CAD build for the part. Positions are in the model's coordinates, mm. A direction names the side the tool comes from. Give positions to 0.01 mm unless a question says otherwise; leave off trailing zeros. Write each loop counter-clockwise with the first axis right and the second up, starting at its lowest first coordinate (ties: lowest second). Pieces come first, ordered by that corner, then holes. Notation, with made-up numbers: (27.25, -2.5) -> (67.25, -2.5) arc R29 cw to (67.25, 20.5) -> close; hole circle Ø9 at (56, 51). An arc over 180 degrees is marked (long way). Use one line per item in the form item = value. Start each with the question number.
from build123d import *

# Parameters (mm, degrees)
BOSS_EXTRUDE1_DEPTH = 20
SKETCH2_R           = 3.25
CUT_EXTRUDE1_DEPTH  = 55.919366752
SKETCH3_R           = 9.1
CUT_EXTRUDE2_DEPTH  = 2
SKETCH4_R           = 1.7
CUT_EXTRUDE3_DEPTH  = 55.919366752
SKETCH5_R           = 1.7
CUT_EXTRUDE4_DEPTH  = 53.677895109
RIB26_REACH         = 46.958
SKETCH15_WALL_W     = 134.175527088
SKETCH15_WALL_H     = 10


with BuildPart() as part:
    # Sketch1 → Boss-Extrude1 (new, symmetric)
    with BuildSketch(Plane(origin=(0, 0, 0), x_dir=(0, 0, -1), z_dir=(1, 0, 0))):
        Polygon((24.929590164, 27.161885246), (24.929590164, -27.838114754), (-29.090409836, -27.838114754), (-29.090409836, -14.908114754), (10.909590164, -14.908114754), (10.909590164, 27.161885246), align=None)
    extrude(amount=BOSS_EXTRUDE1_DEPTH, both=True)

    # Sketch2 → Cut-Extrude1 (cut, through all)
    with BuildSketch(Plane(origin=(0, -14.908114754, 0), x_dir=(1, 0, 0), z_dir=(0, 1, 0))):
        with Locations(Location((0, -9.090409836, 0), (0, 0, 270))):
            Circle(SKETCH2_R)
    extrude(amount=-CUT_EXTRUDE1_DEPTH, mode=Mode.SUBTRACT)

    # Sketch3 → Cut-Extrude2 (cut)
    with BuildSketch(Plane(origin=(0, -14.908114754, 0), x_dir=(1, 0, 0), z_dir=(0, 1, 0))):
        with Locations(Location((0, -9.090409836, 0), (0, 0, 270))):
            Circle(SKETCH3_R)
    extrude(amount=-CUT_EXTRUDE2_DEPTH, mode=Mode.SUBTRACT)

    # Sketch4 → Cut-Extrude3 (cut, through all)
    with BuildSketch(Plane(origin=(0, -14.908114754, 0), x_dir=(1, 0, 0), z_dir=(0, 1, 0))):
        with Locations(Location((0, 1.909590164, 0), (0, 0, 270))):
            Circle(SKETCH4_R)
        with Locations(Location((11, -9.090409836, 0), (0, 0, 270))):
            Circle(SKETCH4_R)
        with Locations(Location((0, -20.090409836, 0), (0, 0, 270))):
            Circle(SKETCH4_R)
        with Locations(Location((-11, -9.090409836, 0), (0, 0, 270))):
            Circle(SKETCH4_R)
    extrude(amount=-CUT_EXTRUDE3_DEPTH, mode=Mode.SUBTRACT)

    # Sketch5 → Cut-Extrude4 (cut, through all)
    with BuildSketch(Plane.XY.offset(-10.909590164)):
        with Locations((-10, 16.126885246)):
            Circle(SKETCH5_R)
        with Locations((10, 16.126885246)):
            Circle(SKETCH5_R)
        with Locations((10, -3.873114754)):
            Circle(SKETCH5_R)
        with Locations((-10, -3.873114754)):
            Circle(SKETCH5_R)
    extrude(amount=-CUT_EXTRUDE4_DEPTH, mode=Mode.SUBTRACT)

    # Sketch15 wall → Rib26 (add, up to next)
    with BuildSketch(Plane(origin=(0, 6.126885246, -8.909590164), x_dir=(0, -0.995510349515, 0.094652754886), z_dir=(0, 0.094652754886, 0.995510349515)), mode=Mode.PRIVATE) as rib26_sk1:
        Rectangle(SKETCH15_WALL_W, SKETCH15_WALL_H)
    rib26_tool1 = extrude(rib26_sk1.sketch, amount=-RIB26_REACH, mode=Mode.PRIVATE) - part.part
    add(rib26_tool1.solids().sort_by_distance((0, 6.126885246, -8.909590164))[0])


solid = part.part
1) 3-axis set-ups, long thin cutter, end or side, ignore diameter. For faces 4 (the face through (-12.03, -21.28, 7.74)), 5 (the face through (13, 6, -10.91)), 6 (the face through (-12, 6, -10.91)), 7 (the face through (-4, -16.908, 9)), 8 (the face through (0, -27.838, 2)): which of +Z, -Z, +X, -X, +Y, -Y reach the whole face in a straight line?
2) Cut at B-B (z = 21). Give the cut face in (x, y).
3) Cut at C-C (y = -21.5). Give the cut face in (x, z), and give its area (3 significant figures).
4) Two-plate mould, pull along X, no slides. Class faces 1 (the face through (0, 0, -24.93)), 2 (the face through (9.779, 17.812, -17.821)), 3 (the face through (-5, 2, -10)): released by +X, released by -X, zero draft, split by the parting line, or undercut.
5) Cut at D-D (z = -16). Give the cut face in (x, y).
6) Wall check: line 1 along Y through (x, z) = (10.5, 16); line 2 along Y through (x, z) = (8, 12); line 3 along Z through (x, y) = (-3, -24.5). Give the ranges that are in metal, low to high. Write a range as from..to.
7) Cut at A-A (x = 0). Give the cut face in (y, z), and give its area (3 significant figures).
8) Pin check, flat tips, straight feed: pin 1 (3 mm diameter, centred on y = 10, z = -9, fed in from -X); pin 2 (4.5 mm diameter, centred on x = 10, y = 16.13, fed in from +Z); pin 3 (14.5 mm diameter, centred on x = 4, z = 7, fed in from +Y). Stop position of each tip, or through.
Final values:
q1.face_4 = +Y, -Y
q1.face_5 = +Z, +X, +Y
q1.face_6 = +Z, -X, +Y
q1.face_7 = +Y
q1.face_8 = +Z, -Z, +X, -X, -Y
q2.outline = (-20, -27.84) -> (-1.44, -27.84) -> (-1.44, -14.91) -> (-20, -14.91) -> close; (1.44, -27.84) -> (20, -27.84) -> (20, -14.91) -> (1.44, -14.91) -> close
q3.outline = (-20, -24.93) -> (20, -24.93) -> (20, 29.09) -> (-20, 29.09) -> close; hole circle Ø3.4 at (-11, 9.09); hole circle Ø6.5 at (0, 9.09); hole circle Ø3.4 at (0, -1.91); hole circle Ø3.4 at (0, 20.09); hole circle Ø3.4 at (11, 9.09)
q3.area = 2,090 mm^2
q4.face_1 = zero draft
q4.face_2 = undercut
q4.face_3 = released by -X
q5.outline = (-20, -27.84) -> (20, -27.84) -> (20, 27.16) -> (-20, 27.16) -> close; hole circle Ø3.4 at (-10, -3.87); hole circle Ø3.4 at (-10, 16.13); hole circle Ø3.4 at (10, -3.87); hole circle Ø3.4 at (10, 16.13)
q6.line_1 = -27.84..-14.91
q6.line_2 = -27.84..-16.91
q6.line_3 = -24.93..7.84, 10.34..29.09
q7.outline = (-27.84, -24.93) -> (27.16, -24.93) -> (27.16, -10.91) -> (-14.91, -6.91) -> (-14.91, -3.61) -> (-27.84, -3.61) -> close; (-27.84, -0.21) -> (-14.91, -0.21) -> (-14.91, -0.01) -> (-16.91, -0.01) -> (-16.91, 5.84) -> (-27.84, 5.84) -> close; (-27.84, 12.34) -> (-16.91, 12.34) -> (-16.91, 18.19) -> (-14.91, 18.19) -> (-14.91, 18.39) -> (-27.84, 18.39) -> close; (-27.84, 21.79) -> (-14.91, 21.79) -> (-14.91, 29.09) -> (-27.84, 29.09) -> close
q7.area = 1,180 mm^2
q8.pin_1 = -5
q8.pin_2 = -10.91
q8.pin_3 = -14.91
